```python
from build123d import *

# Parameters (mm, degrees)
F0_W     = 14
F0_H     = 22.5
F0_R     = 1.75
F1_DEPTH = 4
F2_R     = 1
F3_W     = 1
F3_H     = 6
F4_DEPTH = 0.75
F5_R     = 0.49999


# Not quite as in the source:
# - a fillet or chamfer is up to 0.001 mm smaller than in the source, because OpenCascade refuses the exact size


with BuildPart() as f1:
    # F0 (on Top) → F1 (new body)
    with BuildSketch(Plane.XY):
        with Locations((7, -11.25)):
            Rectangle(F0_W, F0_H)
        with Locations((7, -16)):
            Circle(F0_R, mode=Mode.SUBTRACT)
        with Locations((7, -6.5)):
            Circle(F0_R, mode=Mode.SUBTRACT)
    extrude(amount=F1_DEPTH)

    # F2
    f2_edges = [f1.edges().sort_by_distance(p)[0] for p in [
        (7, 0, 4),
        (0, -11.25, 4),
        (14, -11.25, 4),
        (7, -22.5, 4),
    ]]
    fillet(f2_edges, radius=F2_R)

    # F3 (on face) → F4 (join)
    with BuildSketch(Plane(origin=(0, 0, 0), x_dir=(1, 0, 0), z_dir=(0, 0, -1))):
        with Locations((4, 11.25)):
            Rectangle(F3_W, F3_H)
        with Locations((6, 11.25)):
            Rectangle(F3_W, F3_H)
        with Locations((8, 11.25)):
            Rectangle(F3_W, F3_H)
        with Locations((10, 11.25)):
            Rectangle(F3_W, F3_H)
    extrude(amount=F4_DEPTH)

    # F5 (radius 0.5 in the source; OpenCascade refuses exactly that, so slightly less here)
    f5_edges = [f1.edges().sort_by_distance(p)[0] for p in [
        (10, -8.25, -0.75),
        (10.5, -11.25, -0.75),
        (10, -14.25, -0.75),
        (9.5, -11.25, -0.75),
        (8, -8.25, -0.75),
        (8.5, -11.25, -0.75),
        (8, -14.25, -0.75),
        (7.5, -11.25, -0.75),
        (6, -8.25, -0.75),
        (6.5, -11.25, -0.75),
        (6, -14.25, -0.75),
        (5.5, -11.25, -0.75),
        (4, -8.25, -0.75),
        (4.5, -11.25, -0.75),
        (4, -14.25, -0.75),
        (3.5, -11.25, -0.75),
    ]]
    fillet(f5_edges, radius=F5_R)


solid = f1.part
```
For this review, take the finished solid that the model builds, in its own axes (mm). Give positions to 0.01 mm unless a question says otherwise; leave off trailing zeros. Write each loop counter-clockwise with the first axis right and the second up, starting at its lowest first coordinate (ties: lowest second). Pieces come first, ordered by that corner, then holes. Notation, with made-up numbers: M -7.75,45 L 40.25,45 A30 ccw 40.25,81 Z; hole C 71.5,13 d1. An arc over 180 degrees is marked long. Answer as CSV lines item,"result".
1. Wall thickness on line 1 (Y direction, x = 7, z = 2.05); line 2 (Y direction, x = 6.25, z = 1.85); line 3 (Z direction, x = 8.25, y = -18): over which ranges is each line inside the solid? List them lowest first.
Findings:
line 1,"y = -22.5 to -17.75, -14.25 to -8.25, -4.75 to 0"
line 2,"y = -22.5 to -17.58, -14.42 to -8.08, -4.92 to 0"
line 3,"z = 0 to 4"
2. Consider section C-C, the plane z = 1. Write out the cut boundary in (x, y).
Findings:
outline,"M 0,-22.5 L 14,-22.5 L 14,0 L 0,0 Z; hole C 7,-16 d3.5; hole C 7,-6.5 d3.5"
3. Consider section B-B, the plane y = -16. Write out the cut boundary in (x, z), then the cut area to 3 significant figures.
Findings:
outline,"M 0,0 L 5.25,0 L 5.25,4 L 1,4 A1 ccw 0,3 Z; M 8.75,0 L 14,0 L 14,3 A1 ccw 13,4 L 8.75,4 Z"
area,"41.6 mm2"
4. Draft analysis for pull direction Y (two halves, no side actions). For faces 1 (the flat face through (7, 0, 1)), 2 (the flat face through (7, -22.5, 1)), 3 (the cylindrical face through (6.772, -14.265, 1.972)), 4 (the flat face through (14, -11, 1)), state which applies: +Y half, -Y half, draft (parallel to the pull), parting line (faces both ways), or undercut.
Findings:
face 1,"+Y half"
face 2,"-Y half"
face 3,"undercut"
face 4,"draft"
5. Consider section A-A, the plane x = 7. Write out the cut boundary in (y, z).
Findings:
outline,"M -22.5,0 L -17.75,0 L -17.75,4 L -21.5,4 A1 ccw -22.5,3 Z; M -14.25,0 L -8.25,0 L -8.25,4 L -14.25,4 Z; M -4.75,0 L 0,0 L 0,3 A1 ccw -1,4 L -4.75,4 Z"
